Geometry check sheet. Reference: drawing and pictorial views, mm from the part's lowest x, y, z. Round coordinates to 2 decimals unless told otherwise and drop trailing zeros. Loops run counter-clockwise (first coordinate to the right, second up) from the corner with the lowest first, then second, coordinate; pieces in that order, holes last. Notation, with made-up numbers: (34.5, -33) -> (73.5, -33) arc R4 ccw to (73.5, -26) -> close; hole circle Ø4 at (8, 17.5). An arc over 180 degrees is marked (long way). Use one line per item in the form item = value.
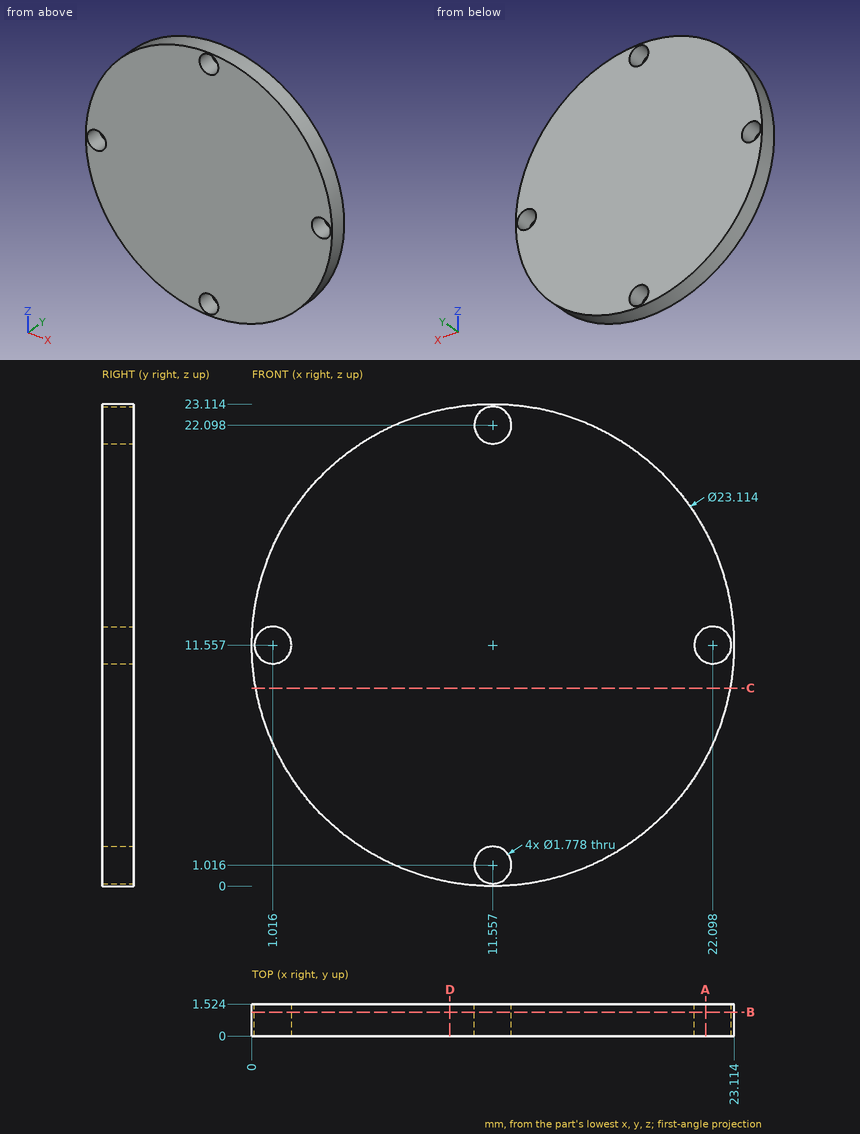
1. Gauge pin test, flat end, axial feed: pin 1 (3 mm diameter, centred on x = 12, z = 9.5, fed in from -Y). Record the tip position at first contact, or that the pin passes through.
Return value:
pin_1 = 0
2. Section check A-A (x = 21.75). Record the boundary of the cut face in (y, z), then the cut area to 3 significant figures.
Return value:
outline = (0, 6.11) -> (1.52, 6.11) -> (1.52, 10.74) -> (0, 10.74) -> close; (0, 12.38) -> (1.52, 12.38) -> (1.52, 17) -> (0, 17) -> close
area = 14.1 mm2
3. Section check B-B (y = 1.15). Record the boundary of the cut face in (x, z) (3 decimals).
Return value:
outline = circle Ø23.114 at (11.557, 11.557); hole circle Ø1.778 at (1.016, 11.557); hole circle Ø1.778 at (11.557, 1.016); hole circle Ø1.778 at (11.557, 22.098); hole circle Ø1.778 at (22.098, 11.557)
4. Section check D-D (x = 9.5). Record the boundary of the cut face in (y, z).
Return value:
outline = (0, 0.18) -> (1.52, 0.18) -> (1.52, 22.93) -> (0, 22.93) -> close
5. Material ranges on line 1 along Z through (x, y) = (11, 0.6); line 2 along Z through (x, y) = (1, 0.75); line 3 along X through (y, z) = (0.9, 10.75), recorded low to high.
Return value:
line_1 = 0.01 to 0.32, 1.71 to 21.41, 22.79 to 23.1
line_2 = 6.85 to 10.67, 12.45 to 16.26
line_3 = 0.03 to 0.64, 1.39 to 21.73, 22.47 to 23.09
6. Section check C-C (z = 9.5). Record the boundary of the cut face in (x, y).
Return value:
outline = (0.18, 0) -> (22.93, 0) -> (22.93, 1.52) -> (0.18, 1.52) -> close
